Design review of the part built by this model. Coordinates are the model's own, in mm. A direction names the side the tool comes from. Give positions to 0.01 mm unless a question says otherwise; leave off trailing zeros. Loops run counter-clockwise (first coordinate to the right, second up) from the corner with the lowest first, then second, coordinate; pieces in that order, holes last. Notation, with made-up numbers: (33.25, -20.5) -> (58.25, -20.5) arc R34 ccw to (58.25, 9.5) -> close; hole circle Ø1 at (64, -1). An arc over 180 degrees is marked (long way). Answer in a Markdown table with one row per item. Add a question column.
(1) Consider section B-B on z = 0. Write out the cut boundary in (x, y).
(2) For faces 1 (the cylindrical face through (-0.54, 2.96, -2.44)), 2 (the flat face through (0, 5.3, 0)), list the 3-axis set-ups (+Z, -Z, +X, -X, +Y, -Y) from which the entire face can be reached by the end or side of a thin tool; tool diameter is ignored.
(3) Consider section D-D on x = 3.25. Write out the cut boundary in (y, z), then the cut area to 3 significant figures.
(4) For line 1 (Y direction, x = 3.25, z = -0.4); line 2 (X direction, y = -6.5, z = 0.8); line 3 (Y direction, x = 0, z = 0.5), list the stretches that pass through material, from the lowest coordinate up.
(5) Consider section A-A on x = 0. Write out the cut boundary in (y, z).
(6) Consider section C-C on y = -0.25. Write out the cut boundary in (x, z), then the cut area to 3 significant figures.
(7) For pin 1 (1.5 mm diameter, centred on y = -16.5, z = -1.5, fed in from -X); pin 2 (1.5 mm diameter, centred on x = 2.5, z = 1.5, fed in from -Y); pin 3 (1 mm diameter, centred on x = 1, y = 0.5, fed in from -Z), all flat-tipped, find the tip position at first contact; note any pin that passes through.
Autodesk Inventor part; units mm, degrees
ref_plane "YZ Plane" through (0, 0, 0) normal (1, 0, 0) x (0, 1, 0)
ref_plane "XZ Plane" through (0, 0, 0) normal (0, 1, 0) x (-1, 0, 0)
ref_plane "XY Plane" through (0, 0, 0) normal (0, 0, 1) x (1, 0, 0)
sketch "Sketch1" plane through (0, 0, 0) normal (0, 1, 0) x (-1, 0, 0)
  arc A0 (-2.958, -0.5) -> (-2.958, 0.5) centre (0, 0) ccw
  line L0 (-3.5, 0) -> (-3.5, -0.5)
  line L1 (-3.5, -0.5) -> (-3, -0.5)
  line L2 (-3, -0.5) -> (-2.958, -0.5)
  line L3 (-3.5, 0) -> (-3.5, 0.5)
  line L4 (-3.5, 0.5) -> (-2.958, 0.5)
  dimension "d0" = 6
  dimension "d1" = 0.5
  dimension "d2" = 0.5
  dimension "d3" = 0.5
extrude "Extrusion1" add sketch "Sketch1" along normal blind 0.2
sketch "Sketch2" plane through (0, 0.2, 0) normal (0, 1, 0) x (1, 0, 0)
  circle A0 centre (0, 0) radius 2.9999
extrude "Extrusion2" add sketch "Sketch2" along normal blind 0.1
sketch "Sketch3" plane through (0, 0.3, 0) normal (0, 1, 0) x (1, 0, 0)
  circle A0 centre (0, 0) radius 2.5
  dimension "d8" = 5
extrude "Extrusion3" add sketch "Sketch3" along normal blind 5
fillet "Fillet1" radius 0.5 1 edges at (-2.5, 5.3, 0)
fillet "Fillet2" radius 1 1 edges at (-2.5, 0.3, 0)
sketch "Sketch4" plane through (0, 0, 0) normal (0, -1, 0) x (1, 0, 0)
  circle A0 centre (0, 0) radius 1.25
  circle A1 centre (0.8555, -0.9113) radius 0.25
  circle A2 centre (0.8555, 0.9113) radius 0.25
  circle A3 centre (-0.8555, -0.9113) radius 0.25
  circle A4 centre (-0.8555, 0.9113) radius 0.25
  dimension "d13" = 2.5
  dimension "d14" = 0.5
  dimension "d16" = 0.5
  dimension "d17" = 0.5
  dimension "d18" = 0.5
extrude "Extrusion4" add sketch "Sketch4" along normal blind 20 contours A2 A0 | A0 A2 | A4 A0 | A0 A4 | A3 A0 | A0 A3
equation "\"BendRadius\" = Thickness"
equation "\"BendReliefWidth\" = Thickness"
equation "\"BendReliefDepth\" = 0.5 * Thickness"
equation "\"CornerReliefSize\" = 4 * Thickness"
equation "\"MinimumRemnant\" = 2 * Thickness"
equation "\"TransitionRadius\" = BendRadius"
equation "\"JacobiRadiusSize\" = BendRadius"
equation "\"GapSize\" = Thickness"
Values follow:
| question | item | result |
|---|---|---|
| 1 | outline | (-3, 0) -> (3.5, 0) -> (3.5, 0.2) -> (3, 0.2) -> (3, 0.3) arc R1 cw to (2.5, 1.17) -> (2.5, 4.8) arc R0.5 ccw to (2, 5.3) -> (-2, 5.3) arc R0.5 ccw to (-2.5, 4.8) -> (-2.5, 1.17) arc R1 cw to (-3, 0.3) -> close |
| 2 | face 1 | +Y |
| 2 | face 2 | +Z, -Z, +X, -X, +Y |
| 3 | outline | (0, -0.5) -> (0.2, -0.5) -> (0.2, 0.5) -> (0, 0.5) -> close |
| 3 | area | 0.200 mm2 |
| 4 | line 1 | 0 to 0.2 |
| 4 | line 2 | -1.08 to -0.63, 0.63 to 1.08 |
| 4 | line 3 | 0 to 5.3 |
| 5 | outline | (0, -3) -> (0.3, -3) arc R1 cw to (1.17, -2.5) -> (4.8, -2.5) arc R0.5 ccw to (5.3, -2) -> (5.3, 2) arc R0.5 ccw to (4.8, 2.5) -> (1.17, 2.5) arc R1 cw to (0.3, 3) -> (0, 3) -> close |
| 6 | outline | circle Ø0.5 at (-0.86, -0.91); circle Ø0.5 at (-0.86, 0.91); circle Ø0.5 at (0.86, 0.91) |
| 6 | area | 0.589 mm2 |
| 7 | pin 1 | x = -1.11 |
| 7 | pin 2 | y = 0 |
| 7 | pin 3 | z = -2.95 |
